Check sheet for the drawn part. Datum: minimum x, y, z corner. Units: mm. A direction names the side the tool comes from. Round coordinates to 2 decimals unless told otherwise and drop trailing zeros. Order: outer loops, then holes, each group sorted by start corner. A loop starts at its lowest first (then second) coordinate and runs counter-clockwise, first axis right, second up. Notation, with made-up numbers: (-11.75, 83.5) -> (7.25, 83.5) arc R32 ccw to (7.25, 119.5) -> close; hole circle Ø6 at (36.25, -36.5). An arc over 180 degrees is marked (long way). Answer in a Markdown table with one row per item.
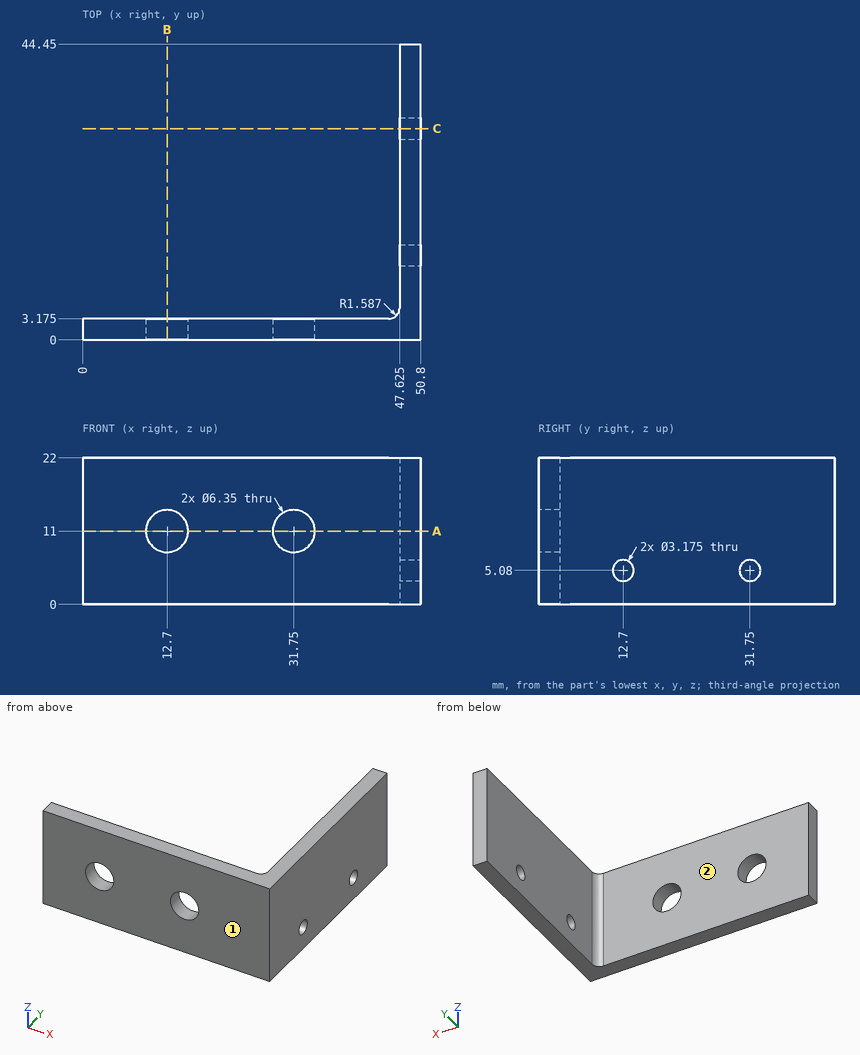
(1) Section check A-A on z = 11. Give the number of separate pieces and of enclosed holes in the cut face.
Solutions:
| item | result |
|---|---|
| separate pieces | 3 |
| enclosed holes | 0 |
(2) Scan lines: probe 1 along Y at (x, z) = (48.35, 5.08); probe 2 along Z at (x, y) = (31.75, 2.4) (1 decimal); probe 3 along Z at (x, y) = (48, 12.5) (1 decimal). Record each from-to range of solid material in increasing order. Write a range as from..to.
Solutions:
| item | result |
|---|---|
| probe 1 | 0..11.11, 14.29..30.16, 33.34..44.45 |
| probe 2 | 0..7.8, 14.2..22 |
| probe 3 | 0..3.5, 6.7..22 |
(3) Section check B-B on x = 12.7. Record the boundary of the cut face in (y, z) (1 decimal).
Solutions:
| item | result |
|---|---|
| outline | (0, 0) -> (3.2, 0) -> (3.2, 7.8) -> (0, 7.8) -> close; (0, 14.2) -> (3.2, 14.2) -> (3.2, 22) -> (0, 22) -> close |
(4) Section check C-C on y = 31.75. Record the boundary of the cut face in (x, z) (1 decimal).
Solutions:
| item | result |
|---|---|
| outline | (47.6, 0) -> (50.8, 0) -> (50.8, 3.5) -> (47.6, 3.5) -> close; (47.6, 6.7) -> (50.8, 6.7) -> (50.8, 22) -> (47.6, 22) -> close |
(5) Tool access check on the marked faces 1 and 2. Record the directions out of +Z, -Z, +X, -X, +Y, -Y that give a thin tool (end or side, any length) a straight path to the whole face; none if there is none.
Solutions:
| item | result |
|---|---|
| face 1 | +Z, -Z, +X, -X, -Y |
| face 2 | +Z, -Z, -X, +Y |
(6) Depth check by flat-ended pin: pin 1 Ø7.5 at (x, z) = (12.7, 11) entering from -Y; pin 2 Ø2.5 at (y, z) = (31.75, 5.08) entering from -X; pin 3 Ø11 at (x, z) = (19, 14.5) entering from +Y (1 decimal); pin 4 Ø3 at (y, z) = (21.5, 13.5) entering from -X (1 decimal). Enter the tip coordinate at first touch or a pass-through.
Solutions:
| item | result |
|---|---|
| pin 1 | y = 0 |
| pin 2 | through |
| pin 3 | y = 3.2 |
| pin 4 | x = 47.6 |
